from build123d import *

# Parameters (mm, degrees)
PAD005_DEPTH = 4
FILLET004_R  = 3
PAD006_DEPTH = 4
FILLET_R     = 3


with BuildPart() as fillet004:
    # Sketch010 → Pad005 (new body)
    with BuildSketch(Plane.XZ.offset(9)):
        Polygon((36.01236, 27.938416), (43.326587, 25.132718), (19.335825, -40.794858), (12.021599, -37.98916), align=None)
    extrude(amount=PAD005_DEPTH)

    # Fillet004
    fillet004_edges = [fillet004.edges().sort_by_distance(p)[0] for p in [
        (36.01236, -11, 27.938416),
        (43.326587, -11, 25.132718),
        (19.335825, -11, -40.794858),
        (12.021599, -11, -37.98916),
    ]]
    fillet(fillet004_edges, radius=FILLET004_R)


with BuildPart() as fusion009:
    # Sketch009 → Pad006 (new body)
    with BuildSketch(Plane.XZ.offset(9)):
        Polygon((-15.121457, 38.064293), (-11.496716, 45.897909), (43.898232, 24.848332), (40.273491, 17.014716), align=None)
    extrude(amount=PAD006_DEPTH)

    # Fillet
    fillet_edges = [fusion009.edges().sort_by_distance(p)[0] for p in [
        (-15.121457, -11, 38.064293),
        (-11.496716, -11, 45.897909),
        (43.898232, -11, 24.848332),
        (40.273491, -11, 17.014716),
    ]]
    fillet(fillet_edges, radius=FILLET_R)

    # Fusion009: union Fillet004
    add(fillet004.part)


solid = fusion009.part
Design review of the part built by this model. Coordinates are the model's own, in mm. A direction names the side the tool comes from. Round coordinates to 2 decimals unless told otherwise and drop trailing zeros. Write each loop counter-clockwise with the first axis right and the second up, starting at its lowest first coordinate (ties: lowest second). Pieces come first, ordered by that corner, then holes. Notation, with made-up numbers: (22, -5.75) - (30, -5.75) arc R16 cw to (30, 12.25) - close; hole circle Ø2 at (69.5, 69). An arc over 180 degrees is marked (long way). Use a Markdown table: item, result. Add a question column.
1. Wall thickness on probe 1 along X at (y, z) = (-12.7, -25); probe 2 along X at (y, z) = (-9.5, 7); probe 3 along Z at (x, y) = (-6, -11.7): over which ranges is each line inside the solid? List them lowest first.
2. For faces 1 (the face through (10.78, -10.97, 28.22)), 2 (the face through (18.835, -11.028, -39.616)), list the 3-axis set-ups (+Z, -Z, +X, -X, +Y, -Y) from which the entire face can be reached by the end or side of a thin tool; tool diameter is ignored.
3. Clearance check with flat-ended pins moving along their axes: pin 1 (1 mm diameter, centred on y = -10, z = 24, fed in from +X); pin 2 (1.5 mm diameter, centred on x = 15, y = -12.5, fed in from +Z). State where each tip first meets the part, or that it passes through.
4. We need section D-D (z = -9.5). State the section outline as (x, y) points.
5. We need section A-A (x = 19.5). State the section outline as (y, z) points, then the cut area to 3 significant figures.
6. Mouldability with a two-part tool opening along Z and no side actions: class faces 3 (the face through (42.005, -10.972, 20.757)), 4 (the face through (39.71, -10.97, 26.52)), 5 (the face through (22.9, -11, -8.1)) as +Z half, -Z half, draft (parallel to the pull), parting line (faces both ways), or undercut.
7. We need section C-C (x = 26). State the section outline as (y, z) points.
8. We need section B-B (y = -12.1). State the section outline as (x, z) points.
Output:
| question | item | result |
|---|---|---|
| 1 | probe 1 | x = 16.75 to 25.08 |
| 1 | probe 2 | x = 28.39 to 36.73 |
| 1 | probe 3 | z = 34.6 to 43.81 |
| 2 | face 1 | -X, +Y, -Y |
| 2 | face 2 | -Z, +Y, -Y |
| 3 | pin 1 | stops at x = 42.81 |
| 3 | pin 2 | stops at z = 36.11 |
| 4 | outline | (22.39, -13) - (30.72, -13) - (30.72, -9) - (22.39, -9) - close |
| 5 | outline | (-13, -39.19) - (-9, -39.19) - (-9, -17.44) - (-13, -17.44) - close; (-13, 24.91) - (-9, 24.91) - (-9, 34.12) - (-13, 34.12) - close |
| 5 | area | 124 mm2 |
| 6 | face 3 | -Z half |
| 6 | face 4 | +Z half |
| 6 | face 5 | undercut |
| 7 | outline | (-13, -22.48) - (-9, -22.48) - (-9, 0.42) - (-13, 0.42) - close; (-13, 22.44) - (-9, 22.44) - (-9, 31.65) - (-13, 31.65) - close |
| 8 | outline | (-13.77, 40.99) arc R3 ccw to (-12.11, 36.92) - (33.04, 19.76) - (13.03, -35.22) arc R3 ccw to (14.77, -39.05) - (16.49, -39.7) arc R3 ccw to (20.38, -37.93) - (41.08, 18.95) arc R3 ccw to (41.45, 19.55) - (42.55, 21.93) arc R3 ccw to (41.23, 25.84) arc R3 ccw to (40.57, 26.19) - (38.86, 26.85) arc R3 ccw to (38.19, 27.02) - (-8.88, 44.9) arc R3 ccw to (-12.67, 43.36) - close |
